Autodesk Inventor part; units mm, degrees
ref_plane "YZ Plane" through (0, 0, 0) normal (1, 0, 0) x (0, 1, 0)
ref_plane "XZ Plane" through (0, 0, 0) normal (0, 1, 0) x (-1, 0, 0)
ref_plane "XY Plane" through (0, 0, 0) normal (0, 0, 1) x (1, 0, 0)
sketch "スケッチ1" plane through (0, 0, 0) normal (1, 0, 0) x (0, 1, 0)
  line L0 (-12.85, 22.85) -> (12.85, 22.85)
  line L1 (12.85, 22.85) -> (12.85, -22.85)
  line L2 (12.85, -22.85) -> (-12.85, -22.85)
  line L3 (-12.85, -22.85) -> (-12.85, 22.85)
  line L4 (-12.85, 22.85) -> (12.85, -22.85) construction
  line L5 (12.85, 22.85) -> (-12.85, -22.85) construction
  line L6 (16.85, -26.85) -> (16.85, 26.85)
  line L7 (16.85, 26.85) -> (-16.85, 26.85)
  line L8 (-16.85, 26.85) -> (-16.85, -26.85)
  line L9 (-16.85, -26.85) -> (16.85, -26.85)
  line L10 (-10, 14.85) -> (10, 14.85)
  line L11 (10, 14.85) -> (10, 38.85)
  line L12 (10, 38.85) -> (-10, 38.85)
  line L13 (-10, 38.85) -> (-10, 14.85)
  line L14 (-10, 14.85) -> (10, 38.85) construction
  line L15 (10, 14.85) -> (-10, 38.85) construction
  line L16 (-10, -14.85) -> (10, -14.85)
  line L17 (10, -14.85) -> (10, -38.85)
  line L18 (10, -38.85) -> (-10, -38.85)
  line L19 (-10, -38.85) -> (-10, -14.85)
  line L20 (-10, -14.85) -> (10, -38.85) construction
  line L21 (10, -14.85) -> (-10, -38.85) construction
  point P0 (0, 0)
  point P1 (0, 26.85)
  point P2 (0, -26.85)
  point P3 (10, -26.85)
  point P4 (-10, -26.85)
  point P5 (-10, 26.85)
  point P6 (10, 26.85)
  dimension "d0" = 25.7
  dimension "d1" = 45.7
  dimension "d2" = 4
  dimension "d5" = 12
  dimension "d6" = 12
  dimension "d7" = 20
  dimension "d8" = 20
extrude "押し出し1" add sketch "スケッチ1" along normal blind 2.5 contours L3 L2 L19 L9 L8 L7 L13 L0 | L13 L7 L11 L0 | L11 L7 L6 L9 L17 L2 L1 L0 | L13 L12 L11 L7 | L2 L17 L9 L19 | L9 L17 L18 L19
fillet "フィレット1" radius 2 8 edges at (1.25, 12.85, 22.85) (1.25, 12.85, -22.85) (1.25, -12.85, -22.85) (1.25, -12.85, 22.85) (1.25, -16.85, 26.85) (1.25, 16.85, 26.85) (1.25, -16.85, -26.85) (1.25, 16.85, -26.85)
fillet "フィレット2" radius 1.5 8 edges at (1.25, 10, 26.85) (1.25, 10, 38.85) (1.25, -10, 38.85) (1.25, -10, 26.85) (1.25, -10, -26.85) (1.25, -10, -38.85) (1.25, 10, -26.85) (1.25, 10, -38.85)
equation "\"d6\" = d5"
equation "\"d8\" = d7"
properties part number "GRS104_hygrometer_fixture_3D プリント"
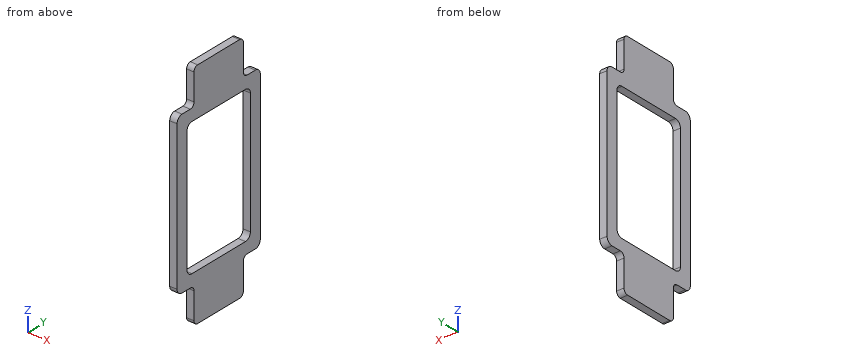
Verification items for the finished model (mm, model axes). Round coordinates to 2 decimals unless told otherwise and drop trailing zeros. Loops run counter-clockwise (first coordinate to the right, second up) from the corner with the lowest first, then second, coordinate; pieces in that order, holes last. Notation, with made-up numbers: (38.5, 22) -> (73.5, 22) arc R24 ccw to (73.5, 58) -> close; hole circle Ø8 at (-2.5, 49.25). An arc over 180 degrees is marked (long way). Answer as a JSON object with one key per item and string values.
Q1. Scan lines: line 1 (Y direction, x = 0.6, z = -20.5); line 2 (Z direction, x = 0.85, y = 2); line 3 (Z direction, x = 0.8, y = -14.5). Record each from-to range of solid material in increasing order. Write a range as from..to.
Data:
{"line 1": "y = -16.85..-12.85, 12.85..16.85", "line 2": "z = -38.85..-22.85, 22.85..38.85", "line 3": "z = -26.85..26.85"}
Q2. Section check A-A (z = -14). Record the boundary of the cut face in (x, y).
Data:
{"outline": "(0, -16.85) -> (2.5, -16.85) -> (2.5, -12.85) -> (0, -12.85) -> close; (0, 12.85) -> (2.5, 12.85) -> (2.5, 16.85) -> (0, 16.85) -> close"}
Q3. Section check D-D (z = -33). Record the boundary of the cut face in (x, y), then the cut area to 3 significant figures.
Data:
{"outline": "(0, -10) -> (2.5, -10) -> (2.5, 10) -> (0, 10) -> close", "area": "50.0 mm2"}
Q4. Go/stop test with flat-tipped pins: P1, Ø1.2, axis at x = 1, y = -12.5, coming from the -Z side; P2, Ø0.8, axis at x = 1.5, y = -13, coming from the +Z side; P3, Ø1.2, axis at x = 1, z = 31.5, coming from the -Y side. Record where each tip stops, or that it passes through.
Data:
{"P1": "stops at z = -26.85", "P2": "stops at z = 26.85", "P3": "stops at y = -10"}
Q5. Section check C-C (y = -5). Record the boundary of the cut face in (x, z), then the cut area to 3 significant figures.
Data:
{"outline": "(0, -38.85) -> (2.5, -38.85) -> (2.5, -22.85) -> (0, -22.85) -> close; (0, 22.85) -> (2.5, 22.85) -> (2.5, 38.85) -> (0, 38.85) -> close", "area": "80.0 mm2"}
